Solid Edge part; units mm, degrees
sketch "Sketch1" plane through (60.3162, 60.3162, 0) normal (0, 0, 1) x (1, 0, 0)
  line L0 (-70.3162, -63.3162) -> (-50.3162, -63.3162)
  line L1 (-50.3162, -63.3162) -> (-50.3162, -57.3162)
  line L2 (-50.3162, -57.3162) -> (-70.3162, -57.3162)
  line L3 (-70.3162, -57.3162) -> (-70.3162, -63.3162)
extrude "Protrusion1" add sketch "Sketch1" along normal blind 300
fillet "Verrundung_1" radius 7.5 2 edges at (-10, 0, 300) (10, 0, 300)
fillet "Verrundung_2" radius 7.5 2 edges at (-10, 0, 0) (10, 0, 0)
hole "Bohrung_1" at (0, -3, 292.5) direction (0, 1, 0) diameter 8 end up to next
hole "Bohrung_2" at (0, -3, 212.5) direction (0, 1, 0) diameter 2.459 end up to next thread major 3 thread length 10
hole "Hole1" at (0, -3, 197.5) direction (0, 1, 0) diameter 2.459 end up to next thread major 3 thread length 10
hole "Hole2" at (0, -3, 182.5) direction (0, 1, 0) diameter 2.459 end up to next thread major 3 thread length 10
hole "Bohrung_5" at (10, 0, 292.5) direction (-1, 0, 0) diameter 2.013 end up to next thread major 2.5 thread length 8
properties material "Aluminium, 1060"
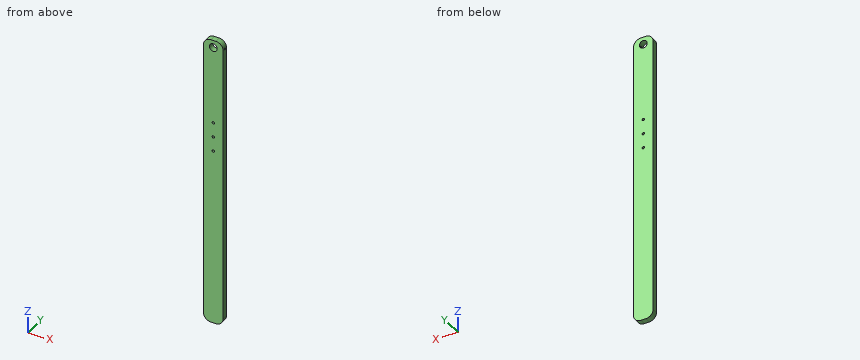
For this review, take the finished solid that the model builds, in its own axes (mm). Coordinates: 2 decimals unless noted, no trailing zeros. Write each loop counter-clockwise with the first axis right and the second up, starting at its lowest first coordinate (ties: lowest second). Pieces come first, ordered by that corner, then holes.
(1) Wall thickness on probe 1 along Z at (x, y) = (0, -0.75); probe 2 along X at (y, z) = (1.5, 292.5); probe 3 along X at (y, z) = (1.55, 212.5): over which ranges is each line inside the solid? List them lowest first.
(2) Add section A-A on y = 0. Give the boundary of the cut face in (x, z), then the cut area to 3 significant figures.
(3) For pin 1 Ø3 at (x, z) = (0, 182.5) entering from -Y; pin 2 Ø2 at (x, y) = (4, 0) entering from +Z, all flat-tipped, find the tip position at first contact; note any pin that passes through.
Answer sheet:
1. probe 1: z = 0 to 181.27, 183.73 to 196.27, 198.73 to 211.27, 213.73 to 288.5, 296.5 to 300
1. probe 2: x = -10 to -4, 4 to 10
1. probe 3: x = -10 to -1.23, 1.23 to 10
2. outline: (-10, 7.5) arc R7.5 ccw to (-2.5, 0) - (2.5, 0) arc R7.5 ccw to (10, 7.5) - (10, 291.49) - (3.87, 291.49) arc R4 cw (long way) to (3.87, 293.51) - (9.93, 293.51) arc R7.5 ccw to (2.5, 300) - (-2.5, 300) arc R7.5 ccw to (-10, 292.5) - close; hole circle Ø2.46 at (0, 182.5); hole circle Ø2.46 at (0, 197.5); hole circle Ø2.46 at (0, 212.5)
2. area: 5,880 mm2
3. pin 1: stops at y = -3
3. pin 2: stops at z = 299.98
